Geometry: final body of the model. Coordinates: model frame, mm. Round coordinates to 2 decimals unless told otherwise and drop trailing zeros. Loops run counter-clockwise (first coordinate to the right, second up) from the corner with the lowest first, then second, coordinate; pieces in that order, holes last. Notation, with made-up numbers: (63.25, -18) -> (103.25, -18) arc R15 cw to (103.25, -2) -> close; hole circle Ø3 at (-9, 52). An arc over 180 degrees is marked (long way). Answer in a Markdown table with one row per item.
```python
from build123d import *

# Parameters (mm, degrees)
BOSS_EXTRUDE1_DEPTH = 3.175
CUT_EXTRUDE1_DEPTH  = 223.848706048
SKETCH3_R           = 1.7018
CUT_EXTRUDE2_DEPTH  = 3.175
FILLET1_R           = 3.175
SKETCH4_R           = 11.1125
CUT_EXTRUDE3_DEPTH  = 222.748694977


with BuildPart() as part:
    # Sketch1 → Boss-Extrude1 (new body)
    with BuildSketch(Plane(origin=(0, 0, 0), x_dir=(1, 0, 0), z_dir=(0, 1, 0))):
        Polygon((-97.967388467, 0), (97.967388467, 0), (187.33670933, 98.456981239), (162.886958446, 120.65), (-162.886958446, 120.65), (-187.33670933, 98.456981239), align=None)
    extrude(amount=BOSS_EXTRUDE1_DEPTH)

    # Sketch2 → Cut-Extrude1 (cut, through all)
    with BuildSketch(Plane(origin=(0, 3.175, 0), x_dir=(1, 0, 0), z_dir=(0, 1, 0))):
        with BuildLine():
            Line((-61.2648, 58.039), (-47.0408, 58.039))
            ThreePointArc((-47.0408, 58.039), (-44.79573597, 58.96893597), (-43.8658, 61.214))
            Line((-43.8658, 61.214), (-43.8658, 95.25))
            ThreePointArc((-43.8658, 95.25), (-44.79573597, 97.49506403), (-47.0408, 98.425))
            Line((-47.0408, 98.425), (-61.2648, 98.425))
            ThreePointArc((-61.2648, 98.425), (-63.50986403, 97.49506403), (-64.4398, 95.25))
            Line((-64.4398, 95.25), (-64.4398, 61.214))
            ThreePointArc((-64.4398, 61.214), (-63.50986403, 58.96893597), (-61.2648, 58.039))
        make_face()
        with BuildLine():
            Line((43.8658, 61.214), (43.8658, 95.25))
            ThreePointArc((43.8658, 95.25), (44.79573597, 97.49506403), (47.0408, 98.425))
            Line((47.0408, 98.425), (61.2648, 98.425))
            ThreePointArc((61.2648, 98.425), (63.50986403, 97.49506403), (64.4398, 95.25))
            Line((64.4398, 95.25), (64.4398, 61.214))
            ThreePointArc((64.4398, 61.214), (63.50986403, 58.96893597), (61.2648, 58.039))
            Line((61.2648, 58.039), (47.0408, 58.039))
            ThreePointArc((47.0408, 58.039), (44.79573597, 58.96893597), (43.8658, 61.214))
        make_face()
    extrude(amount=-CUT_EXTRUDE1_DEPTH, mode=Mode.SUBTRACT)

    # Sketch3 → Cut-Extrude2 (cut)
    with BuildSketch(Plane(origin=(0, 3.175, 0), x_dir=(1, 0, 0), z_dir=(0, 1, 0))):
        with Locations(Location((68.5292, 97.536, 0), (0, 0, 270))):
            Circle(SKETCH3_R)
        with Locations(Location((85.9282, 53.1114, 0), (0, 0, 270))):
            Circle(SKETCH3_R)
        with Locations(Location((-85.9282, 53.1114, 0), (0, 0, 270))):
            Circle(SKETCH3_R)
        with Locations(Location((-68.5292, 97.536, 0), (0, 0, 270))):
            Circle(SKETCH3_R)
    extrude(amount=-CUT_EXTRUDE2_DEPTH, mode=Mode.SUBTRACT)

    # Fillet1
    fillet1_edges = [part.edges().sort_by_distance(p)[0] for p in [
        (-187.33670933, 1.5875, -98.456981239),
        (-162.886958446, 1.5875, -120.65),
        (162.886958446, 1.5875, -120.65),
        (187.33670933, 1.5875, -98.456981239),
        (97.967388467, 1.5875, 0),
        (-97.967388467, 1.5875, 0),
    ]]
    fillet(fillet1_edges, radius=FILLET1_R)

    # Sketch4 → Cut-Extrude3 (cut, through all)
    with BuildSketch(Plane(origin=(0, 3.175, 0), x_dir=(1, 0, 0), z_dir=(0, 1, 0))):
        with Locations(Location((114.4778, 93.6625, 0), (0, 0, 270))):
            Circle(SKETCH4_R)
    extrude(amount=-CUT_EXTRUDE3_DEPTH, mode=Mode.SUBTRACT)


solid = part.part
```
Item 1: Section query C-C, the plane y = 1.95. State how many separate pieces and enclosed holes the cut face has, and give its area (3 significant figures).
Ans:
| item | result |
|---|---|
| separate pieces | 1 |
| enclosed holes | 7 |
| area | 33,800 mm2 |
Item 2: First-contact query: P1, Ø1, axis at y = 3, z = -43, coming from the -X side. Flat tip, straight axial feed; report the tip coordinate or a pass-through.
Ans:
| item | result |
|---|---|
| P1 | x = -137.45 |
Item 3: Mould query, pull axis X, two halves, no side actions, for faces 1 (the cylindrical face through (125.496, 1.61, -95.109)), 2 (the flat face through (174.54, 1.57, -110.07)), 3 (the flat face through (-3, 0, -61)). Classes: released by +X, released by -X, zero draft, split by the parting line, or undercut.
Ans:
| item | result |
|---|---|
| face 1 | undercut |
| face 2 | released by +X |
| face 3 | zero draft |
Item 4: Section query A-A, the plane x = 51.5. Output: boundary loops of the cut face in (y, z) (3 decimals).
Ans:
| item | result |
|---|---|
| outline | (0, -120.65) -> (3.175, -120.65) -> (3.175, -98.425) -> (0, -98.425) -> close; (0, -58.039) -> (3.175, -58.039) -> (3.175, 0) -> (0, 0) -> close |
Item 5: Ray query, L1, parallel to X at y = 1.7, z = -76; L2, parallel to X at y = 2.4, z = -88; L3, parallel to X at y = 2.8, z = -96.5. Return the intervals inside material, ascending.
Ans:
| item | result |
|---|---|
| L1 | -166.95 to -64.44, -43.87 to 43.87, 64.44 to 166.95 |
| L2 | -177.84 to -64.44, -43.87 to 43.87, 64.44 to 104.92, 124.04 to 177.84 |
| L3 | -185.51 to -69.88, -67.18 to -64.18, -44.12 to 44.12, 64.18 to 67.18, 69.88 to 103.73, 125.22 to 185.51 |
Item 6: Section query B-B, the plane z = -67.5. Output: boundary loops of the cut face in (x, y) (3 decimals), and give its area (3 significant figures).
Ans:
| item | result |
|---|---|
| outline | (-159.237, 0) -> (-64.44, 0) -> (-64.44, 3.175) -> (-159.237, 3.175) -> close; (-43.866, 0) -> (43.866, 0) -> (43.866, 3.175) -> (-43.866, 3.175) -> close; (64.44, 0) -> (159.237, 0) -> (159.237, 3.175) -> (64.44, 3.175) -> close |
| area | 881 mm2 |
Item 7: Section query D-D, the plane z = -27. Output: boundary loops of the cut face in (x, y) (3 decimals).
Ans:
| item | result |
|---|---|
| outline | (-122.475, 0) -> (122.475, 0) -> (122.475, 3.175) -> (-122.475, 3.175) -> close |
